```python
from build123d import *

# Parameters (mm, degrees)
F0_W      = 107.95
F0_H      = 63.5
F1_DEPTH  = 57.15
F3_DEPTH  = 31.75
F4_W      = 63.5
F4_H      = 12.7
F5_DEPTH  = 25.401
F7_DEPTH  = 25.401
F9_DEPTH  = 25.401
F11_DEPTH = 50.801


with BuildPart() as f1:
    # F0 (on Front) → F1 (new body)
    with BuildSketch(Plane.XZ):
        with Locations((53.975, 31.75)):
            Rectangle(F0_W, F0_H)
    extrude(amount=-F1_DEPTH)

    # F2 (on face) → F3 (cut)
    with BuildSketch(Plane.XZ):
        Polygon((0, 63.5), (0, 31.75), (44.45, 31.75), (44.45, 19.05), (57.15, 19.05), (57.15, 12.7), (44.45, 12.7), (44.45, 0), (107.95, 0), (107.95, 63.5), align=None)
    extrude(amount=-F3_DEPTH, mode=Mode.SUBTRACT)

    # F4 (on face) → F5 (cut, through all)
    with BuildSketch(Plane.XZ.offset(-31.75)):
        with Locations((76.2, 6.35)):
            Rectangle(F4_W, F4_H)
    extrude(amount=-F5_DEPTH, mode=Mode.SUBTRACT)

    # F6 (on face) → F7 (cut, through all)
    with BuildSketch(Plane.XZ.offset(-31.75)):
        Polygon((50.8, 63.5), (107.95, 31.75), (107.95, 63.5), align=None)
    extrude(amount=-F7_DEPTH, mode=Mode.SUBTRACT)

    # F8 (on face) → F9 (cut, through all)
    with BuildSketch(Plane.XZ.offset(-31.75)):
        with BuildLine():
            ThreePointArc((12.7, 50.8), (19.05, 44.45), (25.4, 50.8))
            ThreePointArc((25.4, 50.8), (19.05, 57.15), (12.7, 50.8))
        make_face()
    extrude(amount=-F9_DEPTH, mode=Mode.SUBTRACT)

    # F10 (on face) → F11 (cut, through all)
    with BuildSketch(Plane(origin=(0, 0, 12.7), x_dir=(1, 0, 0), z_dir=(0, 0, -1))):
        Polygon((107.95, -57.15), (107.95, -41.275), (88.9, -57.15), align=None)
    extrude(amount=-F11_DEPTH, mode=Mode.SUBTRACT)


solid = f1.part
```
Geometry: final body of the model. Coordinates: model frame, mm. A direction names the side the tool comes from. Round coordinates to 2 decimals unless told otherwise and drop trailing zeros. Order: outer loops, then holes, each group sorted by start corner. A loop starts at its lowest first (then second) coordinate and runs counter-clockwise, first axis right, second up. Notation, with made-up numbers: M 23.5,72 L 45.5,72 A26 cw 45.5,100 Z; hole C 83.5,18 d2. An arc over 180 degrees is marked long. Use one line per item in the form item = value. Start each with the question number.
Q1. Cut plane A-A (x = 19.05). Return loops of the section in (y, z).
Q2. Mould query, pull axis X, two halves, no side actions, for faces 6 (the face through (22.464, 44.272, 56.154)), 7 (the face through (34, 57.15, 32)), 8 (the face through (0, 35, 24)). Classes: +X half, -X half, draft (parallel to the pull), parting line (faces both ways), or undercut.
Q3. Cut plane B-B (z = 50.8). Return loops of the section in (x, y).
Q4. Cut plane D-D (z = 25). Return loops of the section in (x, y) (3 decimals), and give its area (3 significant figures).
Q5. Cut plane C-C (y = 26.5). Return loops of the section in (x, z).
Q6. Access query for faces 1 (the face through (98.56, 49.1, 24.02)), 2 (the face through (44.45, 28, 6)), 3 (the face through (57.15, 16, 16)), 4 (the face through (22, 16, 31.75)), 5 (the face through (44.45, 16, 25)). Directions: +Z, -Z, +X, -X, +Y, -Y. A direction counts if a zero-diameter tool reaches every point of the face in a straight line with its end or side. Return the directions, or none.
Q7. Pin query (flat end, axial travel): pin 1 Ø16 at (x, y) = (15, 14) entering from +Z; pin 2 Ø6.5 at (y, z) = (15, 24) entering from +X; pin 3 Ø17 at (x, y) = (77, 36.5) entering from -Z. Return the tip coordinate at first contact, or that it passes through.
Q8. Material intervals for line 1 (Z direction, x = 19.05, y = 44); line 2 (Y direction, x = 33.5, z = 60); line 3 (X direction, y = 50.5, z = 9.5), sorted ascending. Write a range as [from, to].
Geometry results:
q1.outline = M 0,0 L 57.15,0 L 57.15,44.45 L 31.75,44.45 L 31.75,31.75 L 0,31.75 Z; M 31.75,57.15 L 57.15,57.15 L 57.15,63.5 L 31.75,63.5 Z
q2.face_6 = undercut
q2.face_7 = draft
q2.face_8 = -X half
q3.outline = M 0,31.75 L 12.7,31.75 L 12.7,57.15 L 0,57.15 Z; M 25.4,31.75 L 73.66,31.75 L 73.66,57.15 L 25.4,57.15 Z
q4.outline = M 0,0 L 44.45,0 L 44.45,31.75 L 107.95,31.75 L 107.95,41.275 L 88.9,57.15 L 0,57.15 Z
q4.area = 4,000 mm^2
q5.outline = M 0,0 L 44.45,0 L 44.45,12.7 L 57.15,12.7 L 57.15,19.05 L 44.45,19.05 L 44.45,31.75 L 0,31.75 Z
q6.face_1 = +Z, -Z, +X, +Y
q6.face_2 = -Z, +X, +Y, -Y
q6.face_3 = +Z, -Z, +X, -Y
q6.face_4 = +Z, +X, -X, -Y
q6.face_5 = +Z, +X, -Y
q7.pin_1 = 31.75
q7.pin_2 = 44.45
q7.pin_3 = 12.7
q8.line_1 = [0, 44.45], [57.15, 63.5]
q8.line_2 = [31.75, 57.15]
q8.line_3 = [0, 44.45]
